Input: part model. Units: mm. Frame: model coordinates. Face numbers are marked on the shaded views. A direction names the side the tool comes from. Coordinates: 2 decimals unless noted, no trailing zeros. Write each loop counter-clockwise with the first axis right and the second up, starting at its lowest first coordinate (ties: lowest second). Pieces come first, ordered by that corner, then holes. Notation, with made-up numbers: M -39,-23 L 5,-23 A20 cw 5,-1 Z; hole C -14.75,79.5 d8. An arc over 180 degrees is marked long. Answer as a JSON object with one key per item and string values. Group by question number.
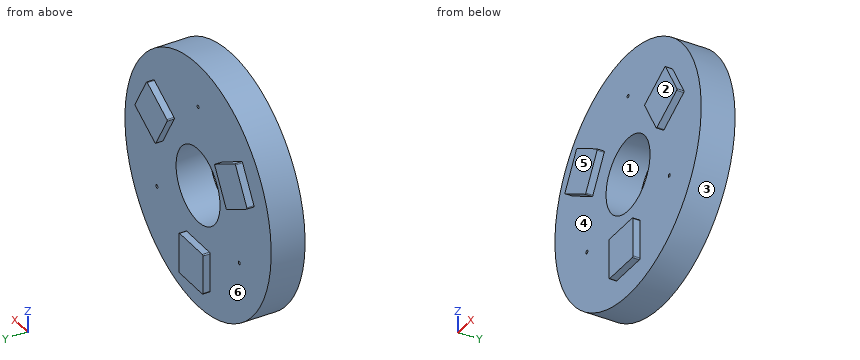
from build123d import *

# Parameters (mm, degrees)
SKETCH1_R            = 18
BOSS_EXTRUDE1_DEPTH  = 2.45505
SKETCH3_R            = 0.238865
SKETCH3_R_2          = 5.4101
CUT_EXTRUDE1_DEPTH   = 26.57395688
CIRPATTERN1_COUNT    = 3
BOSS_EXTRUDE2_DEPTH  = 1.0229375
CIRPATTERN2_COUNT    = 3
MIRROR1_COPY_1_DEPTH = 1.0229375
MIRROR1_COPY_2_DEPTH = 1.0229375


with BuildPart() as part:
    # Sketch1 → Boss-Extrude1 (new, symmetric)
    with BuildSketch(Plane(origin=(0, 0, 0), x_dir=(1, 0, 0), z_dir=(0, 1, 0))):
        with Locations(Location((0, 0, 0), (0, 0, 270))):
            Circle(SKETCH1_R)
    extrude(amount=BOSS_EXTRUDE1_DEPTH, both=True)

    # Sketch3 → Cut-Extrude1 (cut, symmetric)
    with BuildSketch(Plane(origin=(0, 0, 0), x_dir=(1, 0, 0), z_dir=(0, 1, 0))):
        with Locations(Location((0, -11.70505, 0), (0, 0, 270))):
            Circle(SKETCH3_R)
        with Locations(Location((0, 0, 0), (0, 0, 270))):
            Circle(SKETCH3_R_2)
    cut_extrude1 = extrude(amount=CUT_EXTRUDE1_DEPTH, both=True, mode=Mode.SUBTRACT)

    # CirPattern1: Cut-Extrude1 ×3 about axis
    cirpattern1_axis = Axis((0, 0, 0), (0, 1, 0))
    for i in range(1, CIRPATTERN1_COUNT):
        add(cut_extrude1.rotate(cirpattern1_axis, i * 360 / CIRPATTERN1_COUNT), mode=Mode.SUBTRACT)

    # Sketch5 → Boss-Extrude2 (add)
    with BuildSketch(Plane(origin=(0, 2.45505, 0), x_dir=(1, 0, 0), z_dir=(0, 1, 0))):
        with BuildLine():
            Line((-8.871171075, -1.714531368), (-13.698548779, -4.501619185))
            ThreePointArc((-13.698548779, -4.501619185), (-13.774806859, -4.60100065), (-13.758456157, -4.725196563))
            Line((-13.758456157, -4.725196563), (-10.97136834, -9.552574267))
            ThreePointArc((-10.97136834, -9.552574267), (-10.871986875, -9.628832347), (-10.747790962, -9.612481645))
            Line((-10.747790962, -9.612481645), (-5.920413258, -6.825393828))
            ThreePointArc((-5.920413258, -6.825393828), (-5.844155178, -6.726012363), (-5.86050588, -6.60181645))
            Line((-5.86050588, -6.60181645), (-8.647593697, -1.774438746))
            ThreePointArc((-8.647593697, -1.774438746), (-8.746975162, -1.698180666), (-8.871171075, -1.714531368))
        make_face()
    boss_extrude2 = extrude(amount=BOSS_EXTRUDE2_DEPTH)

    # CirPattern2: Boss-Extrude2 ×3 about axis
    cirpattern2_axis = Axis((0, 0, 0), (0, 1, 0))
    for i in range(1, CIRPATTERN2_COUNT):
        add(boss_extrude2.rotate(cirpattern2_axis, i * 360 / CIRPATTERN2_COUNT))

    # Mirror1: Boss-Extrude2 across plane
    add(boss_extrude2.mirror(Plane.ZX))

    # Mirror1 copy 1 sketch → Mirror1 copy 1 (add)
    with BuildSketch(Plane(origin=(0, -2.45505, 0), x_dir=(-0.4999999999999998, 0, -0.8660254037844387), z_dir=(0, -1, 0))):
        with BuildLine():
            Line((-8.871171075, 1.714531368), (-13.698548779, 4.501619185))
            ThreePointArc((-13.698548779, 4.501619185), (-13.774806859, 4.60100065), (-13.758456157, 4.725196563))
            Line((-13.758456157, 4.725196563), (-10.97136834, 9.552574267))
            ThreePointArc((-10.97136834, 9.552574267), (-10.871986875, 9.628832347), (-10.747790962, 9.612481645))
            Line((-10.747790962, 9.612481645), (-5.920413258, 6.825393828))
            ThreePointArc((-5.920413258, 6.825393828), (-5.844155178, 6.726012363), (-5.86050588, 6.60181645))
            Line((-5.86050588, 6.60181645), (-8.647593697, 1.774438746))
            ThreePointArc((-8.647593697, 1.774438746), (-8.746975162, 1.698180666), (-8.871171075, 1.714531368))
        make_face()
    extrude(amount=MIRROR1_COPY_1_DEPTH)

    # Mirror1 copy 2 sketch → Mirror1 copy 2 (add)
    with BuildSketch(Plane(origin=(0, -2.45505, 0), x_dir=(-0.5000000000000004, 0, 0.8660254037844384), z_dir=(0, -1, 0))):
        with BuildLine():
            Line((-8.871171075, 1.714531368), (-13.698548779, 4.501619185))
            ThreePointArc((-13.698548779, 4.501619185), (-13.774806859, 4.60100065), (-13.758456157, 4.725196563))
            Line((-13.758456157, 4.725196563), (-10.97136834, 9.552574267))
            ThreePointArc((-10.97136834, 9.552574267), (-10.871986875, 9.628832347), (-10.747790962, 9.612481645))
            Line((-10.747790962, 9.612481645), (-5.920413258, 6.825393828))
            ThreePointArc((-5.920413258, 6.825393828), (-5.844155178, 6.726012363), (-5.86050588, 6.60181645))
            Line((-5.86050588, 6.60181645), (-8.647593697, 1.774438746))
            ThreePointArc((-8.647593697, 1.774438746), (-8.746975162, 1.698180666), (-8.871171075, 1.714531368))
        make_face()
    extrude(amount=MIRROR1_COPY_2_DEPTH)


solid = part.part
Q1. Section A-A, the plane z = 0. Return the cut outline in (x, y).
Q2. Section B-B, the plane y = -3. Return the cut outline in (x, z), and give its area (3 significant figures).
Q3. Line query: line 1 (Y direction, x = 4, z = 12.5); line 2 (X direction, y = -1.5, z = -1.5); line 3 (Z direction, x = -2, y = 3). Output: solid intervals per line, ascending. Write a range as from..to.
Q4. Section C-C, the plane z = 6. Return the cut outline in (x, y).
Q5. Access query for the marked faces 4, 5 and 6. Directions: +Z, -Z, +X, -X, +Y, -Y. A direction counts if a zero-diameter tool reaches every point of the face in a straight line with its end or side. Return the directions, or none.
Q6. Pin query (flat end, axial travel): pin 1 Ø6.5 at (x, z) = (0, 0) entering from +Y; pin 2 Ø12 at (x, z) = (-11, -8) entering from -Y; pin 3 Ø18 at (x, z) = (7.5, -6) entering from -Y; pin 4 Ø0.8 at (x, y) = (-1, 3) entering from +Z. Return the tip coordinate at first contact, or that it passes through.
Q7. Draft query along X for the marked faces 1, 2 and 3. Return one class per face: released by +X, released by -X, zero draft, split by the parting line, or undercut.
Q8. Section D-D, the plane y = -1. Return the cut outline in (x, z).
Filled in:
{
 "1": {"outline": "M -18,-2.46 L -5.41,-2.46 L -5.41,2.46 L -18,2.46 Z; M 5.41,-2.46 L 18,-2.46 L 18,2.46 L 5.41,2.46 Z"},
 "2": {"outline": "M -13.76,4.73 A0.16 ccw -13.7,4.5 L -8.87,1.71 A0.16 ccw -8.65,1.77 L -5.86,6.6 A0.16 ccw -5.92,6.83 L -10.75,9.61 A0.16 ccw -10.97,9.55 Z; M -2.95,-14.11 A0.16 ccw -2.79,-14.28 L 2.79,-14.28 A0.16 ccw 2.95,-14.11 L 2.95,-8.54 A0.16 ccw 2.79,-8.38 L -2.79,-8.38 A0.16 ccw -2.95,-8.54 Z; M 5.86,6.6 L 8.65,1.77 A0.16 ccw 8.87,1.71 L 13.7,4.5 A0.16 ccw 13.76,4.73 L 10.97,9.55 A0.16 ccw 10.75,9.61 L 5.92,6.83 A0.16 ccw Z", "area": "104 mm^2"},
 "3": {"line 1": "-2.46..2.46", "line 2": "-17.94..-5.2, 5.2..17.94", "line 3": "-14.28..-8.38"},
 "4": {"outline": "M -16.97,-2.46 L -13.02,-2.46 L -13.02,-3.48 L -6.21,-3.48 L -6.21,-2.46 L 6.21,-2.46 L 6.21,-3.48 L 13.02,-3.48 L 13.02,-2.46 L 16.97,-2.46 L 16.97,2.46 L 13.02,2.46 L 13.02,3.48 L 6.21,3.48 L 6.21,2.46 L -6.21,2.46 L -6.21,3.48 L -13.02,3.48 L -13.02,2.46 L -16.97,2.46 Z"},
 "5": {"face 4": "-Y", "face 5": "+Z, -Z, +X, -X, -Y", "face 6": "+Y"},
 "6": {"pin 1": "through", "pin 2": "y = -2.46", "pin 3": "y = -3.48", "pin 4": "z = -8.38"},
 "7": {"face 1": "undercut", "face 2": "zero draft", "face 3": "split by the parting line"},
 "8": {"outline": "C 0,0 d36; hole C -10.14,-5.85 d0.48; hole C 0,0 d10.82; hole C 0,11.71 d0.48; hole C 10.14,-5.85 d0.48"}
}
